```python
from build123d import *

# Parameters (mm, degrees)
SKETCH2_W                 = 8.1026
SKETCH2_H                 = 15.875
CUT_EXTRUDE1_DEPTH        = 509.158439859
FILLET1_R                 = 0.9
CHAMFER1_SIZE             = 0.5
CHAMFER2_SIZE             = 0.68
CHAMFER2_SIZE2            = 0.804519922
M6X1_0_TAPPED_HOLE3_D     = 5
M6X1_0_TAPPED_HOLE3_DEPTH = 14.986
M6X1_0_TAPPED_HOLE3_TIP   = 1.502151548
CUT_EXTRUDE2_DEPTH        = 511.484084003
FILLET9_R                 = 0.6
CHAMFER3_SIZE             = 1
FILLET11_R                = 1.5
CHAMFER4_SIZE             = 0.5
CHAMFER5_SIZE             = 1
CHAMFER6_SIZE             = 1
CHAMFER8_SIZE             = 1
CHAMFER9_SIZE             = 0.5


with BuildPart() as part:
    # Sketch1 → Revolve1 (revolve)
    with BuildSketch(Plane.XY, mode=Mode.PRIVATE) as revolve1_sk:
        Polygon((0, 38.5), (0, 22.225), (57.770884658, 13.8), (71.066827565, 20), (78.696152423, 20), (79.5, 17), (86.5, 17), (86.5, 17.25), (95.732693176, 17.25), (117, 13.5), (170, 13.5), (170, 12.7), (278.5, 12.7), (278.5, 16), (285.5, 16), (285.5, 16.5), (487, 16.5), (487, 17.75), (490, 17.75), (490, 17.5), (499, 17.5), (499, 18), (504, 18), (505, 18.577350269), (505, 27.5), (481.5, 27.5), (481.5, 29), (421.5, 29), (421.5, 28.5), (369, 28.5), (369, 30), (340, 30), (340, 28.4), (172, 28.4), (172, 30), (167, 30), (167, 28.4353), (164.8156, 28.4353), (164.8156, 30), (35, 30), (35, 40), (1.5, 40), align=None)
    revolve(revolve1_sk.sketch.rotate(Axis((-259.751915285, 0, 0), (1, 0, 0)), 90), axis=Axis((-259.751915285, 0, 0), (1, 0, 0)))

    # Sketch2 → Cut-Extrude1 (cut, through all)
    with BuildSketch(Plane.XY):
        with Locations((4.0513, 0)):
            Rectangle(SKETCH2_W, SKETCH2_H)
    extrude(amount=CUT_EXTRUDE1_DEPTH, mode=Mode.SUBTRACT)

    # Fillet1
    fillet1_edges = [part.edges().sort_by_distance(p)[0] for p in [
        (8.1026, -7.9375, 29.346744713),
        (8.1026, 7.9375, 29.346744713),
    ]]
    fillet(fillet1_edges, radius=FILLET1_R)

    # Chamfer1
    chamfer1_edges = [part.edges().sort_by_distance(p)[0] for p in [
        (0, -7.9375, 29.216069478),
        (0, 7.9375, 29.216069478),
    ]]
    chamfer(chamfer1_edges, length=CHAMFER1_SIZE)

    # Chamfer2
    chamfer2_edges = [part.edges().sort_by_distance(p)[0] for p in [
        (0, 0, -22.225),
    ]]
    chamfer2_side = [part.faces().sort_by_distance(p)[0] for p in [
        (0, 0, -23.307346581),
    ]]
    chamfer(chamfer2_edges, length=CHAMFER2_SIZE, length2=CHAMFER2_SIZE2, reference=chamfer2_side[0])

    # M6x1.0 Tapped Hole3
    with Locations(Plane.ZY.offset(-8.1026)):
        with Locations((33.15, 0)):
            Hole(M6X1_0_TAPPED_HOLE3_D / 2, depth=M6X1_0_TAPPED_HOLE3_DEPTH)
            with Locations((0, 0, -(M6X1_0_TAPPED_HOLE3_DEPTH + M6X1_0_TAPPED_HOLE3_TIP / 2))):  # 118° drill point
                Cone(0, M6X1_0_TAPPED_HOLE3_D / 2, M6X1_0_TAPPED_HOLE3_TIP, mode=Mode.SUBTRACT)

    # Sketch5 → Cut-Extrude2 (cut, through all)
    with BuildSketch(Plane.XY.offset(23)):
        with BuildLine():
            Line((429.5, 7), (473.5, 7))
            ThreePointArc((473.5, 7), (480.5, 0), (473.5, -7))
            Line((473.5, -7), (429.5, -7))
            ThreePointArc((429.5, -7), (422.5, 0), (429.5, 7))
        make_face()
    extrude(amount=CUT_EXTRUDE2_DEPTH, mode=Mode.SUBTRACT)

    # Fillet9
    fillet9_edges = [part.edges().sort_by_distance(p)[0] for p in [
        (422.5, 0, 23),
        (451.5, -7, 23),
        (480.5, 0, 23),
        (451.5, 7, 23),
    ]]
    fillet(fillet9_edges, radius=FILLET9_R)

    # Chamfer3
    chamfer3_edges = [part.edges().sort_by_distance(p)[0] for p in [
        (505, 0, -27.5),
    ]]
    chamfer(chamfer3_edges, length=CHAMFER3_SIZE)

    # Fillet11
    fillet11_edges = [part.edges().sort_by_distance(p)[0] for p in [
        (35, 0, -30),
    ]]
    fillet(fillet11_edges, radius=FILLET11_R)

    # Chamfer4
    chamfer4_edges = [part.edges().sort_by_distance(p)[0] for p in [
        (35, 0, -40),
    ]]
    chamfer(chamfer4_edges, length=CHAMFER4_SIZE)

    # Chamfer5
    chamfer5_edges = [part.edges().sort_by_distance(p)[0] for p in [
        (172, 0, -30),
    ]]
    chamfer(chamfer5_edges, length=CHAMFER5_SIZE)

    # Chamfer6
    chamfer6_edges = [part.edges().sort_by_distance(p)[0] for p in [
        (340, 0, -30),
        (369, 0, -30),
    ]]
    chamfer(chamfer6_edges, length=CHAMFER6_SIZE)

    # Chamfer8
    chamfer8_edges = [part.edges().sort_by_distance(p)[0] for p in [
        (481.5, 0, -29),
    ]]
    chamfer(chamfer8_edges, length=CHAMFER8_SIZE)

    # Chamfer9
    chamfer9_edges = [part.edges().sort_by_distance(p)[0] for p in [
        (421.5, 0, -29),
    ]]
    chamfer(chamfer9_edges, length=CHAMFER9_SIZE - 0.0001)  # a hair under: the kernel refuses the full size


solid = part.part
```
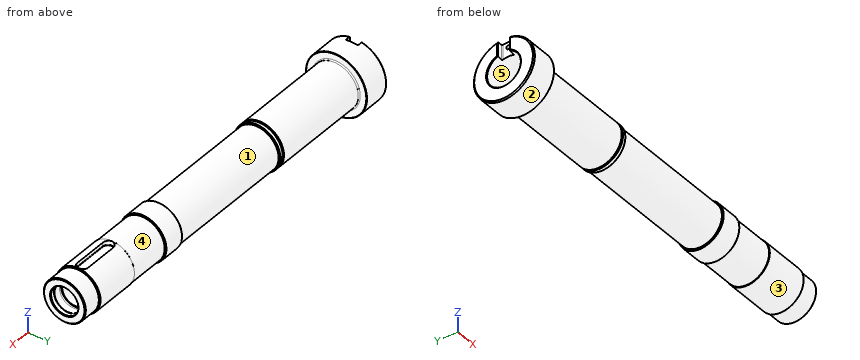
Read the model definition and answer for the solid it produces. Units are mm, in the model's axes. Face numbers are marked on the shaded views. A direction names the side the tool comes from. Coordinates: 2 decimals unless noted, no trailing zeros. Write each loop counter-clockwise with the first axis right and the second up, starting at its lowest first coordinate (ties: lowest second). Pieces come first, ordered by that corner, then holes. Notation, with made-up numbers: (51, 73) - (77, 73) arc R13 ccw to (77, 84) - close; hole circle Ø11 at (37, -1). An arc over 180 degrees is marked (long way). Answer as a JSON object with one key per item and string values. Group by question number.
1. A cutting plane is placed at A-A (x = 444). Determine the outline of the cut face in (y, z).
2. The mould has two halves that part along Z. Classify the marked faces 4 and 5: +Z half, -Z half, draft (parallel to the pull), parting line (faces both ways), or undercut.
3. A cutting plane is placed at B-B (x = 373.5). Determine the outline of the cut face in (y, z), plus the area to 3 significant figures.
4. Consider L1, parallel to Z at x = 268, y = 1; L2, parallel to Y at x = 280, z = 0; L3, parallel to Y at x = 90, z = 0. Determine where each line is inside the solid, lowest interval first. Write a range as [from, to].
5. Each of these flat-tipped pins is pushed along its axis until it touches: P1, Ø6.5, axis at y = 0, z = 33.15, coming from the -X side; P2, Ø2.5, axis at x = 457.5, z = 26.5, coming from the +Y side; P3, Ø6, axis at x = 139, y = 19.5, coming from the +Z side; P4, Ø21.5, axis at y = 0, z = 0, coming from the -X side. Where does it stop, or does it pass through?
6. Which of the six approach directions +Z, -Z, +X, -X, +Y, -Y give full straight-line access (tool end or side, diameter ignored) to the marked faces 1, 2 and 3?
Worked out:
{
 "1": {"outline": "(-7, 23.6) - (-7, 28.14) arc R29 ccw (long way) to (7, 28.14) - (7, 23.6) arc R0.6 cw to (6.4, 23) - (-6.4, 23) arc R0.6 cw to start; hole circle Ø33 at (0, 0)"},
 "2": {"face 4": "parting line", "face 5": "undercut"},
 "3": {"outline": "circle Ø57 at (0, 0); hole circle Ø33 at (0, 0)", "area": "1,700 mm²"},
 "4": {"L1": "z = [-28.38, -12.66], [12.66, 28.38]", "L2": "y = [-28.4, -16], [16, 28.4]", "L3": "y = [-30, -17.25], [17.25, 30]"},
 "5": {"P1": "stops at x = 8.1", "P2": "stops at y = 14.26", "P3": "stops at z = 25.05", "P4": "passes through"},
 "6": {"face 1": "none", "face 2": "+X, -X", "face 3": "+X"}
}
